Could you check a few things on this model? Use its own coordinates, in mm. A direction names the side the tool comes from. Coordinates: 2 decimals unless noted, no trailing zeros. Order: outer loops, then holes, each group sorted by start corner. A loop starts at its lowest first (then second) coordinate and runs counter-clockwise, first axis right, second up. Notation, with made-up numbers: M -26.75,76 L -2.75,76 A16 cw -2.75,83 Z; hole C 82.25,34 d1. An arc over 180 degrees is marked long. Write item = value, one per line. Start each with the question number.
from build123d import *

# Parameters (mm, degrees)
FILLET1_R    = 0.4
RECPAT_COUNT = 2
RECPAT_ANGLE = 90


with BuildPart() as part:
    # BodySke → Base-Revolve (revolve)
    with BuildSketch(Plane.XY, mode=Mode.PRIVATE) as base_revolve_sk:
        with BuildLine():
            Line((4.8, 4), (4.8, 8.9))
            Line((4.8, 8.9), (4.105264982, 8.9))
            ThreePointArc((4.105264982, 8.9), (1.075772976, 4.900591816), (0, 0))
            Line((0, 0), (39.8, 0))
            Line((39.8, 0), (39.8, 4))
            Line((39.8, 4), (4.8, 4))
        make_face()
    revolve(base_revolve_sk.sketch.rotate(Axis((-25.4, 0, 0), (1, 0, 0)), 90), axis=Axis((-25.4, 0, 0), (1, 0, 0)))

    # Fillet1
    fillet1_edges = [part.edges().sort_by_distance(p)[0] for p in [
        (4.8, 0, -4),
    ]]
    fillet(fillet1_edges, radius=FILLET1_R)

    # Sketch3 → Recess section 0
    with BuildSketch(Plane(origin=(0, 0, 0), x_dir=(0, 0, -1), z_dir=(1, 0, 0))):
        with BuildLine():
            Line((0.71, -3.9), (-0.71, -3.9))
            Line((-0.71, -3.9), (-0.71, 3.9))
            Line((-0.71, 3.9), (0.71, 3.9))
            Line((0.71, 3.9), (0.71, -3.9))
        make_face()
    # Sketch4 → Recess section 1
    with BuildSketch(Plane(origin=(4.36, 0, 0), x_dir=(0, 0, -1), z_dir=(1, 0, 0))):
        with BuildLine():
            Line((0.71, -1.726184552), (-0.71, -1.726184552))
            Line((-0.71, -1.726184552), (-0.71, 1.726184552))
            Line((-0.71, 1.726184552), (0.71, 1.726184552))
            Line((0.71, 1.726184552), (0.71, -1.726184552))
        make_face()
    recess = loft(mode=Mode.SUBTRACT)

    # RecPat: Recess ×2 about axis
    recpat_axis = Axis((0, 0, 0), (1, 0, 0))
    for i in range(1, RECPAT_COUNT):
        add(recess.rotate(recpat_axis, i * RECPAT_ANGLE / (RECPAT_COUNT - 1)), mode=Mode.SUBTRACT)

    # RecCorSke → RecessCore (revolve, cut)
    with BuildSketch(Plane.XY, mode=Mode.PRIVATE) as recesscore_sk:
        Polygon((0, 0), (0, 1.5853809), (4.36, 1.2805), (4.776059671, 0), align=None)
    revolve(recesscore_sk.sketch.rotate(Axis((-3.175, 0, 0), (1, 0, 0)), 348.85798225), axis=Axis((-3.175, 0, 0), (1, 0, 0)), mode=Mode.SUBTRACT)


solid = part.part
(1) Imagine slicing it at A-A on x = 10.5. List the corners of the cut face in (y, z) for me.
(2) Please list where these lines run through material, in increasing order: probe 1 along Y at (x, z) = (27, 0.25); probe 2 along Z at (x, y) = (37, -1.75). Write a range as from..to.
(3) Thinking about a two-plate mould opening in Z: for faces 1 (the cylindrical face through (4.448, -6.015, -6.56)), 2 (the flat face through (4.8, -2.1, 4.1)), 3 (the flat face through (2.49, 2.66, 0.01)), which applies, released by +Z, released by -Z, zero draft, split by the parting line, or undercut?
(4) Imagine slicing it at B-B on z = -5.25. List the corners of the cut face in (x, y) for me.
(5) Will these pins go through, and if not, where does the flat tip stop? P1, Ø1.5, axis at x = 21, z = 1, coming from the -Y side; P2, Ø4, axis at y = 4, z = -5.5, coming from the -X side; P3, Ø1.5, axis at x = 25, y = 3.5, coming from the -Z side; P4, Ø8, axis at y = 3.5, z = 1, coming from the -X side.
(6) For faces 4 (the flat face through (39.8, 0, 0)), 5 (the cylindrical face through (22.258, 3.905, -0.867)), 6 (the flat face through (2.49, -2.66, -0.01)), which set-ups out of +Z, -Z, +X, -X, +Y, -Y let a thin tool reach every point of the face, with its end or its side?
Response:
q1.outline = C 0,0 d8
q2.probe_1 = -3.99..3.99
q2.probe_2 = -3.6..3.6
q3.face_1 = split by the parting line
q3.face_2 = zero draft
q3.face_3 = undercut
q4.outline = M 4.11,-7.19 L 4.8,-7.19 L 4.8,7.19 L 4.11,7.19 A10.46 ccw Z
q5.P1 = -3.99
q5.P2 = 1.03
q5.P3 = -2.9
q5.P4 = 0.11
q6.face_4 = +Z, -Z, +X, +Y, -Y
q6.face_5 = +X
q6.face_6 = -X
